from build123d import *

# Parameters (mm, degrees)
F1_DEPTH = 30
F3_R     = 2
F4_DEPTH = 7
F5_R     = 12.5
F6_DEPTH = 7


with BuildPart() as f1:
    # F0 (on Front) → F1 (new body)
    with BuildSketch(Plane.XZ):
        Polygon((15, -21.5), (15, -14.5), (-15, -14.5), (-15, 14.5), (15, 14.5), (15, 21.5), (-22, 21.5), (-22, -21.5), align=None)
    extrude(amount=F1_DEPTH)

    # F3 (on face) → F4 (cut, through all)
    with BuildSketch(Plane(origin=(0, 0, -21.5), x_dir=(1, 0, 0), z_dir=(0, 0, -1))):
        with Locations((8, 23)):
            Circle(F3_R)
        with Locations((8, 7)):
            Circle(F3_R)
    extrude(amount=-F4_DEPTH, mode=Mode.SUBTRACT)

    # F5 (on face) → F6 (cut, through all)
    with BuildSketch(Plane(origin=(-22, 0, 0), x_dir=(0, -1, 0), z_dir=(-1, 0, 0))):
        with Locations((15, 0)):
            Circle(F5_R)
    extrude(amount=-F6_DEPTH, mode=Mode.SUBTRACT)


solid = f1.part
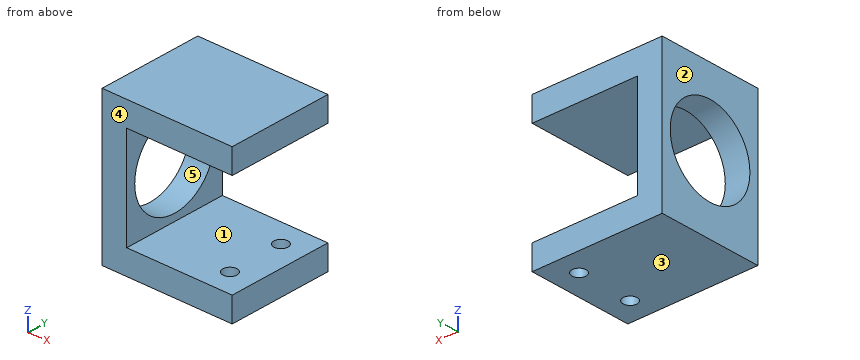
For this review, take the finished solid that the model builds, in its own axes (mm). Face numbers are marked on the shaded views. A direction names the side the tool comes from. Round coordinates to 2 decimals unless told otherwise and drop trailing zeros. Order: outer loops, then holes, each group sorted by start corner. A loop starts at its lowest first (then second) coordinate and runs counter-clockwise, first axis right, second up. Notation, with made-up numbers: (7.5, 53) -> (45.5, 53) arc R25 ccw to (45.5, 69) -> close; hole circle Ø3 at (19, -7.75). An arc over 180 degrees is marked (long way). Put each result on its own line as item: value.
Q1. Add section B-B on z = -10. Write out the cut boundary in (x, y), plus the area to 3 significant figures.
Check result:
outline: (-22, -30) -> (-15, -30) -> (-15, -22.5) -> (-22, -22.5) -> close; (-22, -7.5) -> (-15, -7.5) -> (-15, 0) -> (-22, 0) -> close
area: 105 mm2
Q2. For probe 1 along Y at (x, z) = (8, -16.5); probe 2 along Z at (x, y) = (-2, -27.5); probe 3 along X at (y, z) = (-23, -17.25), list the stretches that pass through material, from the lowest coordinate up. Write a range as [from, to].
Check result:
probe 1: [-30, -25], [-21, -9], [-5, 0]
probe 2: [-21.5, -14.5], [14.5, 21.5]
probe 3: [-22, 6], [10, 15]
Q3. Add section A-A on y = -15. Write out the cut boundary in (x, z).
Check result:
outline: (-22, -21.5) -> (15, -21.5) -> (15, -14.5) -> (-15, -14.5) -> (-15, -12.5) -> (-22, -12.5) -> close; (-22, 12.5) -> (-15, 12.5) -> (-15, 14.5) -> (15, 14.5) -> (15, 21.5) -> (-22, 21.5) -> close
Q4. Machinability: for the marked faces 1 and 2, which of the approach directions +Z, -Z, +X, -X, +Y, -Y give a long, thin tool a straight path to every point of the face, cutting with its end or side? Answer none if there is none.
Check result:
face 1: +X, +Y, -Y
face 2: +Z, -Z, -X, +Y, -Y
Q5. Add section D-D on x = -20. Write out the cut boundary in (y, z), plus the area to 3 significant figures.
Check result:
outline: (-30, -21.5) -> (0, -21.5) -> (0, 21.5) -> (-30, 21.5) -> close; hole circle Ø25 at (-15, 0)
area: 799 mm2
Q6. Add section C-C on x = 8. Write out the cut boundary in (y, z).
Check result:
outline: (-30, -21.5) -> (-25, -21.5) -> (-25, -14.5) -> (-30, -14.5) -> close; (-30, 14.5) -> (0, 14.5) -> (0, 21.5) -> (-30, 21.5) -> close; (-21, -21.5) -> (-9, -21.5) -> (-9, -14.5) -> (-21, -14.5) -> close; (-5, -21.5) -> (0, -21.5) -> (0, -14.5) -> (-5, -14.5) -> close
Q7. Mouldability with a two-part tool opening along Z and no side actions: class the marked faces 3, 4 and 5 as pulls with the +Z half, pulls with the -Z half, needs draft (parallel to the pull), parting line crosses it, or undercut.
Check result:
face 3: pulls with the -Z half
face 4: needs draft
face 5: undercut
Q8. Insertion check: pin 1 Ø8.5 at (y, z) = (-21, -5) entering from +X; pin 2 Ø2 at (y, z) = (-3, -9.5) entering from +X. Each pin has a flat end and moves straight along its axis. Give the tip position at first contact, or say it passes through.
Check result:
pin 1: through
pin 2: x = -15
